Autodesk Fusion 360 part; units mm, degrees
sketch "Sketch1" plane through (0, 0, 0) normal (0, 0, 1) x (1, 0, 0)
  line L0 (0, 0) -> (165, 0)
  line L1 (165, 0) -> (165, 50)
  line L2 (165, 50) -> (0, 50)
  line L3 (0, 50) -> (0, 0)
  line L4 (0, 50) -> (10, 50)
  line L5 (10, 50) -> (10, 0)
  line L6 (10, 0) -> (0, 0)
  line L7 (0, 0) -> (0, 50)
  line L8 (165, 50) -> (155, 50)
  line L9 (155, 50) -> (155, 0)
  line L10 (155, 0) -> (165, 0)
  line L11 (165, 0) -> (165, 50)
  line L12 (0, 10) -> (165, 10)
  line L13 (165, 10) -> (165, 0)
  line L14 (165, 0) -> (0, 0)
  line L15 (0, 0) -> (0, 10)
  dimension "d1" = 165
  dimension "d2" = 50
  dimension "d3" = 10
  dimension "d4" = 10
  dimension "d5" = 50
extrude "Extrude1" add sketch "Sketch1" along normal blind 10 contours L0 L3 L5 L6 L7 L12 L14 L15 | L0 L5 L9 L12 L14 | L2 L3 L4 L5 L7 L12 | L0 L1 L9 L10 L11 L12 L13 L14 | L1 L2 L8 L9 L11 L12
sketch "Sketch2" plane through (0, 0, 10) normal (0, 0, 1) x (-1, 0, 0)
  line L0 (-165, 0) -> (-165, -50)
  line L1 (-165, -50) -> (-155, -50)
  line L2 (-155, -50) -> (-155, -10)
  line L3 (-155, -10) -> (-10, -10)
  line L4 (-10, -10) -> (-10, -50)
  line L5 (-10, -50) -> (0, -50)
  line L6 (0, -50) -> (0, 0)
  line L7 (0, 0) -> (-165, 0)
  circle A0 centre (-5, -45) radius 2
  circle A1 centre (-160, -45) radius 2
  dimension "d8" = 4
  dimension "d9" = 4
extrude "Extrude2" cut sketch "Sketch2" against normal blind 10 contours A0 | A1
sketch "Sketch3" plane through (0, 0, 10) normal (0, 0, 1) x (-1, 0, 0)
  circle A0 centre (-160, -45) radius 2
  circle A1 centre (-5, -45) radius 2
  line L0 (-165, 0) -> (-165, -50)
  line L1 (-165, -50) -> (-155, -50)
  line L2 (-155, -50) -> (-155, -10)
  line L3 (-155, -10) -> (-10, -10)
  line L4 (-10, -10) -> (-10, -50)
  line L5 (-10, -50) -> (0, -50)
  line L6 (0, -50) -> (0, 0)
  line L7 (0, 0) -> (-165, 0)
  line L8 (0, 0) -> (-20, 0)
  line L9 (-20, 0) -> (-25, 0)
  line L10 (-25, 0) -> (-25, -10)
  line L11 (-25, -10) -> (-20, -10)
  line L12 (-20, -10) -> (-20, 0)
  line L13 (-25, 0) -> (-60, 0)
  line L14 (-60, 0) -> (-65, 0)
  line L15 (-65, 0) -> (-65, -10)
  line L16 (-65, -10) -> (-60, -10)
  line L17 (-60, -10) -> (-60, 0)
  line L18 (-65, 0) -> (-100, 0)
  line L19 (-100, 0) -> (-105, 0)
  line L20 (-105, 0) -> (-105, -10)
  line L21 (-105, -10) -> (-100, -10)
  line L22 (-100, -10) -> (-100, 0)
  line L23 (-105, 0) -> (-140, 0)
  line L24 (-140, 0) -> (-145, 0)
  line L25 (-145, 0) -> (-145, -10)
  line L26 (-145, -10) -> (-140, -10)
  line L27 (-140, -10) -> (-140, 0)
  dimension "d12" = 20
  dimension "d13" = 5
  dimension "d14" = 10
  dimension "d15" = 35
  dimension "d16" = 35
  dimension "d17" = 35
extrude "Extrude3" add sketch "Sketch3" along normal blind 25 contours L3 L7 L24 L25 L26 L27 | L3 L7 L19 L20 L21 L22 | L3 L7 L14 L15 L16 L17 | L3 L7 L9 L10 L11 L12
sketch "Sketch4" plane through (0, 10, 0) normal (0, 1, 0) x (-1, 0, 0)
  line L0 (-155, 0) -> (-10, 0)
  line L1 (-10, 0) -> (-10, 10)
  line L2 (-10, 10) -> (-20, 10)
  line L3 (-20, 10) -> (-20, 35)
  line L4 (-20, 35) -> (-25, 35)
  line L5 (-25, 35) -> (-25, 10)
  line L6 (-25, 10) -> (-60, 10)
  line L7 (-60, 10) -> (-60, 35)
  line L8 (-60, 35) -> (-65, 35)
  line L9 (-65, 35) -> (-65, 10)
  line L10 (-65, 10) -> (-100, 10)
  line L11 (-100, 10) -> (-100, 35)
  line L12 (-100, 35) -> (-105, 35)
  line L13 (-105, 35) -> (-105, 10)
  line L14 (-105, 10) -> (-140, 10)
  line L15 (-140, 10) -> (-140, 35)
  line L16 (-140, 35) -> (-145, 35)
  line L17 (-145, 35) -> (-145, 10)
  line L18 (-145, 10) -> (-155, 10)
  line L19 (-155, 10) -> (-155, 0)
  line L20 (-20, 30) -> (-25, 30)
  line L21 (-25, 30) -> (-25, 35)
  line L22 (-25, 35) -> (-20, 35)
  line L23 (-20, 35) -> (-20, 30)
  line L24 (-60, 30) -> (-65, 30)
  line L25 (-65, 30) -> (-65, 35)
  line L26 (-65, 35) -> (-60, 35)
  line L27 (-60, 35) -> (-60, 30)
  line L28 (-100, 30) -> (-105, 30)
  line L29 (-105, 30) -> (-105, 35)
  line L30 (-105, 35) -> (-100, 35)
  line L31 (-100, 35) -> (-100, 30)
  line L32 (-140, 30) -> (-145, 30)
  line L33 (-145, 30) -> (-145, 35)
  line L34 (-145, 35) -> (-140, 35)
  line L35 (-140, 35) -> (-140, 30)
extrude "Extrude4" add sketch "Sketch4" along normal blind 5 contours L15 L16 L17 L32 L33 L34 L35 | L3 L4 L5 L20 L21 L22 L23 | L11 L12 L13 L28 L29 L30 L31 | L7 L8 L9 L24 L25 L26 L27
Input: part model. Units: mm. Frame: model coordinates. A direction names the side the tool comes from. Coordinates: 2 decimals unless noted, no trailing zeros. Write each loop counter-clockwise with the first axis right and the second up, starting at its lowest first coordinate (ties: lowest second). Pieces come first, ordered by that corner, then holes. Notation, with made-up numbers: M 38,26.25 L 95,26.25 A32 cw 95,57.25 Z; hole C 2,8.25 d2. An arc over 180 degrees is marked long. Answer as a JSON object with one key per item and string values. Group by question number.
(1) Ray query, line 1 along X through (y, z) = (45, 3.5); line 2 along Y through (x, z) = (160, 7.5); line 3 along X through (y, z) = (16.5, 5.5). Return the intervals inside material, ascending. Write a range as [from, to].
(2) Section C-C on y = 36.5. Output: boundary loops of the cut face in (x, z), plus the area to 3 significant figures.
(3) Section A-A on z = 16.5. Output: boundary loops of the cut face in (x, y).
(4) Mould query, pull axis Y, two halves, no side actions, for faces 1 (the face through (102, 12, 30)), 2 (the face through (161.6, 46.2, 5.1)), 3 (the face through (160, 50, 5)). Classes: pulls with the +Y half, pulls with the -Y half, needs draft (parallel to the pull), parting line crosses it, or undercut.
(5) Section B-B on x = 5. Output: boundary loops of the cut face in (y, z), plus the area to 3 significant figures.
(6) Set-up query: faces 4 (the face through (155, 30, 5)), 5 (the face through (122, 5, 10)), 6 (the face through (20, 6, 22)). Return all of +Z, -Z, +X, -X, +Y, -Y with unobstructed straight access to the full face (end or side cutting, diameter ignored); none if empty.
(7) Contact query for flat-ended pins moving along their axis: P1, Ø5.5, axis at x = 102, y = 13, coming from the -Z side; P2, Ø5.5, axis at x = 101.5, z = 32, coming from the +Y side; P3, Ø12, axis at x = 139, z = 14.5, coming from the +Y side; P4, Ø8, axis at x = 121, z = 14.5, coming from the +Y side. Output: stop coordinate, or through.
(8) Section D-D on y = 45. Output: boundary loops of the cut face in (x, z).
Result set:
{
 "1": {"line 1": "x = [0, 3], [7, 10], [155, 158], [162, 165]", "line 2": "y = [0, 43], [47, 50]", "line 3": "x = [0, 10], [155, 165]"},
 "2": {"outline": "M 0,0 L 10,0 L 10,10 L 0,10 Z; M 155,0 L 165,0 L 165,10 L 155,10 Z", "area": "200 mm2"},
 "3": {"outline": "M 20,0 L 25,0 L 25,10 L 20,10 Z; M 60,0 L 65,0 L 65,10 L 60,10 Z; M 100,0 L 105,0 L 105,10 L 100,10 Z; M 140,0 L 145,0 L 145,10 L 140,10 Z"},
 "4": {"face 1": "needs draft", "face 2": "undercut", "face 3": "pulls with the +Y half"},
 "5": {"outline": "M 0,0 L 43,0 L 43,10 L 0,10 Z; M 47,0 L 50,0 L 50,10 L 47,10 Z", "area": "460 mm2"},
 "6": {"face 4": "+Z, -Z, +Y", "face 5": "+Z, +Y, -Y", "face 6": "+Z, -X, +Y, -Y"},
 "7": {"P1": "stops at z = 30", "P2": "stops at y = 15", "P3": "stops at y = 10", "P4": "passes through"},
 "8": {"outline": "M 0,0 L 3,0 L 3,10 L 0,10 Z; M 7,0 L 10,0 L 10,10 L 7,10 Z; M 155,0 L 158,0 L 158,10 L 155,10 Z; M 162,0 L 165,0 L 165,10 L 162,10 Z"}
}
